from build123d import *

# Parameters (mm, degrees)
BOSS_EXTRUDE1_DEPTH = 25.4
FILLET1_R           = 12.7
SKETCH2_R           = 7.9375
CUT_EXTRUDE1_DEPTH  = 25.4


with BuildPart() as part:
    # Sketch1 → Boss-Extrude1 (new body)
    with BuildSketch(Plane.XY):
        Polygon((-53.975, 0), (53.975, 0), (53.975, 76.2), (0, 127), (-53.975, 76.2), align=None)
    extrude(amount=BOSS_EXTRUDE1_DEPTH)

    # Fillet1
    fillet1_edges = [part.edges().sort_by_distance(p)[0] for p in [
        (0, 127, 12.7),
    ]]
    fillet(fillet1_edges, radius=FILLET1_R)

    # Sketch2 → Cut-Extrude1 (cut)
    with BuildSketch(Plane.XY.offset(25.4)):
        with Locations((0, 107.95)):
            Circle(SKETCH2_R)
    extrude(amount=-CUT_EXTRUDE1_DEPTH, mode=Mode.SUBTRACT)


solid = part.part
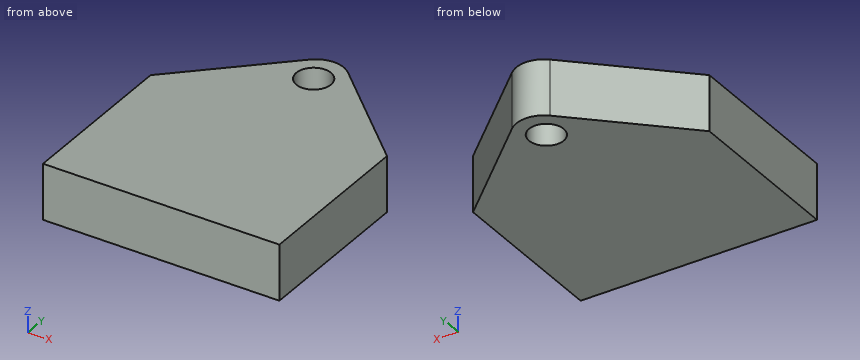
Geometry: final body of the model. Coordinates: model frame, mm. Coordinates: 2 decimals unless noted, no trailing zeros. Order: outer loops, then holes, each group sorted by start corner. A loop starts at its lowest first (then second) coordinate and runs counter-clockwise, first axis right, second up. Notation, with made-up numbers: M 9,-5.5 L 63,-5.5 A7 ccw 63,3.5 Z; hole C 53,-39 d10. An arc over 180 degrees is marked long. One line per question, with ' | ' between items. Start each with the question number.
Item 1: Cut plane A-A, the plane x = 0. Return the cut outline in (y, z), then the cut area to 3 significant figures.
Item 2: Ray query, probe 1 along Y at (x, z) = (0, 17); probe 2 along Y at (x, z) = (2, 10.75); probe 3 along Y at (x, z) = (33, 2.5). Return the intervals inside material, ascending. Write a range as [from, to].
Item 3: Cut plane B-B, the plane y = 107.95. Return the cut outline in (x, z), then the cut area to 3 significant figures.
Item 4: Pin query (flat end, axial travel): pin 1 Ø2 at (y, z) = (86.5, 4) entering from -X. Return the tip coordinate at first contact, or that it passes through.
Item 5: Cut plane D-D, the plane y = 83. Return the cut outline in (x, z), then the cut area to 3 significant figures.
A:
1) outline: M 0,0 L 100.01,0 L 100.01,25.4 L 0,25.4 Z; M 115.89,0 L 122.26,0 L 122.26,25.4 L 115.89,25.4 Z | area: 2,700 mm2
2) probe 1: y = [0, 100.01], [115.89, 122.26] | probe 2: y = [0, 100.27], [115.63, 122.1] | probe 3: y = [0, 95.94]
3) outline: M -20.24,0 L -7.94,0 L -7.94,25.4 L -20.24,25.4 Z; M 7.94,0 L 20.24,0 L 20.24,25.4 L 7.94,25.4 Z | area: 625 mm2
4) pin 1: stops at x = -44.09
5) outline: M -46.75,0 L 46.75,0 L 46.75,25.4 L -46.75,25.4 Z | area: 2,370 mm2
